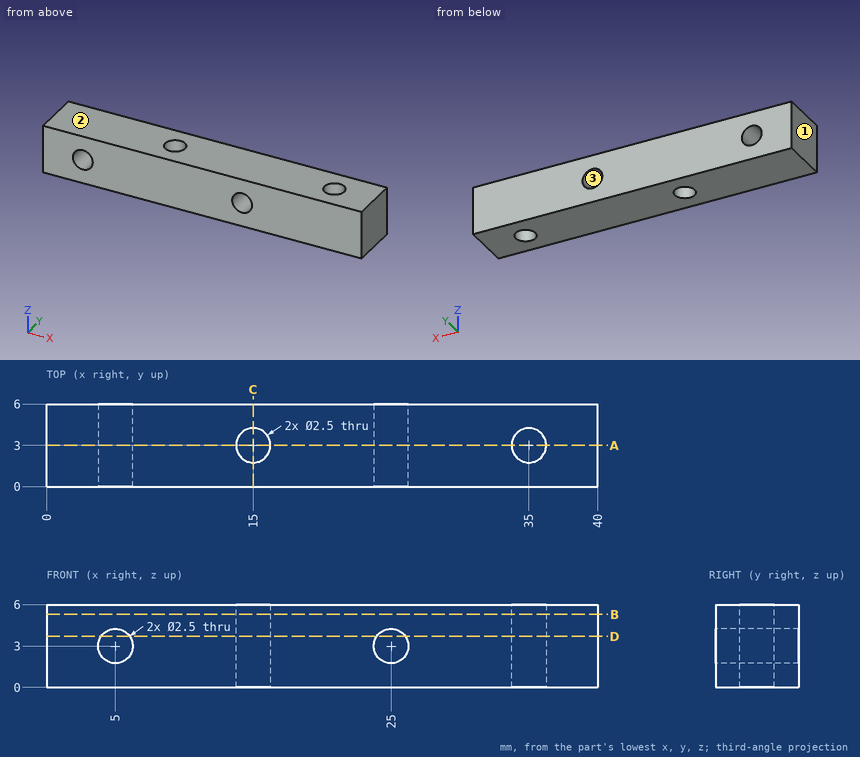
Could you check a few things on this drawing? It's one solid part, dimensions in mm from its lowest x, y, z. Round coordinates to 2 decimals unless told otherwise and drop trailing zeros. Order: outer loops, then holes, each group sorted by start corner. A loop starts at its lowest first (then second) coordinate and runs counter-clockwise, first axis right, second up. Notation, with made-up numbers: M 83,70 L 114,70 A17 cw 114,74 Z; hole C 58,22 d8. An arc over 180 degrees is marked long. Use a Markdown table: item, result.
1) Imagine slicing it at A-A (y = 3). List the corners of the cut face in (x, z) for me.
Geometry says:
| item | result |
|---|---|
| outline | M 0,0 L 13.75,0 L 13.75,6 L 0,6 Z; M 16.25,0 L 33.75,0 L 33.75,6 L 16.25,6 Z; M 36.25,0 L 40,0 L 40,6 L 36.25,6 Z; hole C 5,3 d2.5; hole C 25,3 d2.5 |
2) Imagine slicing it at C-C (x = 15). List the corners of the cut face in (y, z) for me, then the cut area to 3 significant figures.
Geometry says:
| item | result |
|---|---|
| outline | M 0,0 L 1.75,0 L 1.75,6 L 0,6 Z; M 4.25,0 L 6,0 L 6,6 L 4.25,6 Z |
| area | 21.0 mm² |
3) If we mould it in two halves opening along Z, with no side actions, what happens to the marked faces 1, 2 and 3? For each: +Z half, -Z half, draft (parallel to the pull), parting line (faces both ways), or undercut.
Geometry says:
| item | result |
|---|---|
| face 1 | draft |
| face 2 | +Z half |
| face 3 | undercut |
4) Imagine slicing it at D-D (z = 3.7). List the corners of the cut face in (x, y) for me, then the cut area to 3 significant figures.
Geometry says:
| item | result |
|---|---|
| outline | M 0,0 L 3.96,0 L 3.96,6 L 0,6 Z; M 6.04,0 L 23.96,0 L 23.96,6 L 6.04,6 Z; M 26.04,0 L 40,0 L 40,6 L 26.04,6 Z; hole C 15,3 d2.5; hole C 35,3 d2.5 |
| area | 205 mm² |
5) If I drill on line 1 along X through (y, z) = (2.9, 3); line 2 along Y through (x, z) = (15, 2.2); line 3 along X through (y, z) = (0.5, 2.95), over which ranges is the centre line in solid material (lowest first)?
Geometry says:
| item | result |
|---|---|
| line 1 | x = 0 to 3.75, 6.25 to 13.75, 16.25 to 23.75, 26.25 to 33.75, 36.25 to 40 |
| line 2 | y = 0 to 1.75, 4.25 to 6 |
| line 3 | x = 0 to 3.75, 6.25 to 23.75, 26.25 to 40 |
6) Imagine slicing it at B-B (z = 5.3). List the corners of the cut face in (x, y) for me.
Geometry says:
| item | result |
|---|---|
| outline | M 0,0 L 40,0 L 40,6 L 0,6 Z; hole C 15,3 d2.5; hole C 35,3 d2.5 |
